Part model, mm, in its own coordinate system. A direction names the side the tool comes from. Give positions to 0.01 mm unless a question says otherwise; leave off trailing zeros. Order: outer loops, then holes, each group sorted by start corner. A loop starts at its lowest first (then second) coordinate and runs counter-clockwise, first axis right, second up. Notation, with made-up numbers: (50.5, 13.5) -> (56.5, 13.5) arc R20 cw to (56.5, 51.5) -> close; hole circle Ø3 at (34.5, 8). An arc over 180 degrees is marked (long way). Write item = value, one per line. Start each with the question number.
Item 1: Flat gauge pins, fed straight in: P1, Ø20, axis at x = 50, y = 36.5, coming from the +Z side; P2, Ø5, axis at x = 71, y = 24, coming from the -Z side; P3, Ø2.5, axis at x = 4, y = 54, coming from the -Z side; P4, Ø1.5, axis at x = 74.5, y = 13.5, coming from the +Z side. Where does each tip first touch, or does it go through?
Item 2: Band-saw the part on D-D on x = 64.5. Write the cut outline in (y, z).
Item 3: Band-saw the part on B-B on y = 4. Write the cut outline in (x, z).
Item 4: Tool access for faces 3 (the face through (43, 4, 8)), 4 (the face through (29.9, 15, 4)): list every direction of +Z, -Z, +X, -X, +Y, -Y with a clear straight run to the whole face (end or side of a thin tool).
Item 5: Drill centre lines: line 1 along X through (y, z) = (10, 7.25); line 2 along Y through (x, z) = (24, 4); line 3 along Y through (x, z) = (13.9, 3.6). Where is each one in solid material? Low to high.
Item 6: Band-saw the part on A-A on x = 84. Write the cut outline in (y, z).
Item 7: Band-saw the part on C-C on z = 4.5. Count the separate pieces of the cut face and the enclosed holes in it, plus the area to 3 significant figures.
Item 8: Pull direction X, two halves, no side cores. Call faces 1 (the face through (43, 0, 4)), 2 (the face through (40, 45.1, 4)): +X half, -X half, draft (parallel to the pull), parting line (faces both ways), or undercut.
```python
from build123d import *

# Parameters (mm, degrees)
SKETCH_2_W          = 88
SKETCH_2_H          = 58
SKETCH_2_R          = 1.55
EXTRUDE_4_DEPTH     = 8
SKETCH_6_W          = 70.2
SKETCH_6_H          = 40.2
CUT_EXTRUDE_4_DEPTH = 2
SKETCH_7_R          = 1.5
SKETCH_7_W          = 10
SKETCH_7_H          = 7
SKETCH_7_W_2        = 7
SKETCH_7_H_2        = 10
SKETCH_7_W_3        = 11.2
SKETCH_7_H_3        = 8
CUT_EXTRUDE_7_DEPTH = 5


with BuildPart() as part:
    # 草图2 → 凸台-拉伸4 (new body)
    with BuildSketch(Plane.XY):
        with Locations((44, 29)):
            Rectangle(SKETCH_2_W, SKETCH_2_H)
        with Locations((4, 4)):
            Circle(SKETCH_2_R, mode=Mode.SUBTRACT)
        with Locations(Location((4, 54, 0), (0, 0, 180))):
            Circle(SKETCH_2_R, mode=Mode.SUBTRACT)
        with Locations(Location((84, 4, 0), (0, 0, 180))):
            Circle(SKETCH_2_R, mode=Mode.SUBTRACT)
        with Locations((84, 54)):
            Circle(SKETCH_2_R, mode=Mode.SUBTRACT)
    extrude(amount=EXTRUDE_4_DEPTH)

    # 草图6 → 切除-拉伸4 (cut)
    with BuildSketch(Plane.XY.offset(8)):
        with Locations((44, 29)):
            Rectangle(SKETCH_6_W, SKETCH_6_H)
    extrude(amount=-CUT_EXTRUDE_4_DEPTH, mode=Mode.SUBTRACT)

    # 草图7 → 切除-拉伸7 (cut)
    with BuildSketch(Plane.XY.offset(6)):
        with Locations((13.9, 13.9)):
            Circle(SKETCH_7_R)
        with Locations(Location((14, 44, 0), (0, 0, 180))):
            Circle(SKETCH_7_R)
        with Locations(Location((74.1, 13.9, 0), (0, 0, 180))):
            Circle(SKETCH_7_R)
        with Locations((74, 44)):
            Circle(SKETCH_7_R)
        with Locations((24.9, 15.4)):
            Rectangle(SKETCH_7_W, SKETCH_7_H)
        with Locations((72.6, 33.1)):
            Rectangle(SKETCH_7_W_2, SKETCH_7_H_2)
        with Locations((40.5, 41.1)):
            Rectangle(SKETCH_7_W_3, SKETCH_7_H_3)
    extrude(amount=-CUT_EXTRUDE_7_DEPTH, mode=Mode.SUBTRACT)


solid = part.part
```
Values found:
q1.P1 = 6
q1.P2 = 0
q1.P3 = through
q1.P4 = 1
q2.outline = (0, 0) -> (58, 0) -> (58, 8) -> (49.1, 8) -> (49.1, 6) -> (8.9, 6) -> (8.9, 8) -> (0, 8) -> close
q3.outline = (0, 0) -> (2.45, 0) -> (2.45, 8) -> (0, 8) -> close; (5.55, 0) -> (82.45, 0) -> (82.45, 8) -> (5.55, 8) -> close; (85.55, 0) -> (88, 0) -> (88, 8) -> (85.55, 8) -> close
q4.face_3 = +Z, +X, -X, +Y, -Y
q4.face_4 = +Z
q5.line_1 = 0 to 8.9, 79.1 to 88
q5.line_2 = 0 to 11.9, 18.9 to 58
q5.line_3 = 0 to 12.4, 15.4 to 42.5, 45.5 to 58
q6.outline = (0, 0) -> (2.45, 0) -> (2.45, 8) -> (0, 8) -> close; (5.55, 0) -> (52.45, 0) -> (52.45, 8) -> (5.55, 8) -> close; (55.55, 0) -> (58, 0) -> (58, 8) -> (55.55, 8) -> close
q7.separate_pieces = 1
q7.enclosed_holes = 11
q7.area = 4,820 mm^2
q8.face_1 = draft
q8.face_2 = undercut
